Check sheet for the modelled part. Datum: model origin and axes. Units: mm. A direction names the side the tool comes from. Give positions to 0.01 mm unless a question says otherwise; leave off trailing zeros. Write each loop counter-clockwise with the first axis right and the second up, starting at its lowest first coordinate (ties: lowest second). Pieces come first, ordered by that corner, then holes. Notation, with made-up numbers: (6, -2.75) -> (18, -2.75) arc R34 ccw to (18, 31.25) -> close; hole circle Ø2 at (-31.75, -33.75). An arc over 180 degrees is marked (long way). Write each question's results on one line, items separated by ' | '. Start each with the question number.
Autodesk Inventor part; units mm, degrees
ref_plane "YZ Plane" through (0, 0, 0) normal (1, 0, 0) x (0, 1, 0)
ref_plane "XZ Plane" through (0, 0, 0) normal (0, 1, 0) x (-1, 0, 0)
ref_plane "XY Plane" through (0, 0, 0) normal (0, 0, 1) x (1, 0, 0)
sketch "Sketch1" plane through (0, 0, 0) normal (0, 0, 1) x (1, 0, 0)
  line L0 (0, 0) -> (-112.5, 0) construction
  line L1 (-112.5, 0) -> (112.5, 0) construction
  line L2 (0, 0) -> (0, 100) construction
  line L3 (0, 100) -> (0, -100) construction
  line L4 (0, 0) -> (-75, 0) construction
  line L5 (-75, 0) -> (-75, -55) construction
  line L6 (0, 0) -> (75, 0) construction
  line L7 (75, 0) -> (75, -55) construction
  arc A0 (-72.2813, -59.7687) -> (72.2813, -59.7687) centre (0, -15.4013) ccw
  line L8 (-112.5, 0) -> (-112.5, -45)
  line L9 (-102.5, -55) -> (-80.8039, -55)
  line L10 (80.8039, -55) -> (102.5, -55)
  line L11 (112.5, -45) -> (112.5, 0)
  line L12 (-75, 0) -> (-75, 55) construction
  line L13 (75, 0) -> (75, 55) construction
  arc A1 (72.2746, 59.7368) -> (-72.2746, 59.7368) centre (0, 15) ccw
  line L14 (-80.7775, 55) -> (-102.5, 55)
  line L15 (-112.5, 45) -> (-112.5, 0)
  line L16 (80.7775, 55) -> (102.5, 55)
  line L17 (112.5, 45) -> (112.5, 0)
  arc A2 (-102.5, 55) -> (-112.5, 45) centre (-102.5, 45) ccw
  arc A3 (-80.7775, 55) -> (-72.2746, 59.7368) centre (-80.7775, 65) ccw
  arc A4 (72.2746, 59.7368) -> (80.7775, 55) centre (80.7775, 65) ccw
  arc A5 (112.5, 45) -> (102.5, 55) centre (102.5, 45) ccw
  arc A6 (102.5, -55) -> (112.5, -45) centre (102.5, -45) ccw
  arc A7 (80.8039, -55) -> (72.2813, -59.7687) centre (80.8039, -65) ccw
  arc A8 (-72.2813, -59.7687) -> (-80.8039, -55) centre (-80.8039, -65) ccw
  arc A9 (-112.5, -45) -> (-102.5, -55) centre (-102.5, -45) ccw
  line L18 (-72.2746, 59.7368) -> (-61.9878, 53.5577) construction
  line L19 (-61.9878, 53.5577) -> (-58.8982, 58.7011)
  line L20 (-58.8982, 58.7011) -> (-33.1812, 43.2534)
  line L21 (-33.1812, 43.2534) -> (-36.2707, 38.11)
  line L22 (-36.2707, 38.11) -> (-61.9878, 53.5577)
  line L23 (-58.8982, 58.7011) -> (-56.8385, 62.1301)
  line L24 (-56.8385, 62.1301) -> (-31.1215, 46.6823)
  line L25 (-31.1215, 46.6823) -> (-28.0319, 51.8257)
  line L26 (-28.0319, 51.8257) -> (-53.749, 67.2735)
  line L27 (-53.749, 67.2735) -> (-56.8385, 62.1301)
  line L28 (75.9108, 56.2641) -> (66.1713, 49.254) construction
  line L29 (66.1713, 49.254) -> (62.6662, 54.1238) construction
  line L30 (62.6662, 54.1238) -> (38.3174, 36.5986) construction
  line L31 (38.3174, 36.5986) -> (41.8224, 31.7289) construction
  line L32 (41.8224, 31.7289) -> (66.1713, 49.254) construction
  line L33 (62.6662, 54.1238) -> (56.8245, 62.2401) construction
  line L34 (56.8245, 62.2401) -> (60.3296, 57.3703) construction
  line L35 (60.3296, 57.3703) -> (35.9829, 39.842) construction
  line L36 (35.9829, 39.842) -> (32.4779, 44.7118) construction
  line L37 (32.4779, 44.7118) -> (56.8245, 62.2401) construction
  line L38 (-75, -55) -> (-66.4238, -46.6067) construction
  line L39 (-66.4238, -46.6067) -> (-55.2326, -58.0416) construction
  line L40 (-55.2326, -58.0416) -> (-59.4293, -53.7535) construction
  line L41 (-59.4293, -53.7535) -> (-37.9887, -32.7702) construction
  line L42 (-37.9887, -32.7702) -> (-33.792, -37.0583) construction
  line L43 (-55.2326, -58.0416) -> (-33.792, -37.0583) construction
  line L44 (-66.4238, -46.6067) -> (-62.2271, -50.8948) construction
  line L45 (-62.2271, -50.8948) -> (-40.7865, -29.9114) construction
  line L46 (-40.7865, -29.9114) -> (-44.9832, -25.6233) construction
  line L47 (-44.9832, -25.6233) -> (-66.4238, -46.6067) construction
  line L48 (66.1713, -50.8948) -> (57.2172, -64.1547) construction
  line L49 (57.2172, -64.1547) -> (60.3546, -59.0403) construction
  line L50 (60.3546, -59.0403) -> (34.7828, -43.3533) construction
  line L51 (34.7828, -43.3533) -> (31.6454, -48.4676) construction
  line L52 (57.2172, -64.1547) -> (31.6454, -48.4676) construction
  line L53 (66.1713, -50.8948) -> (62.8135, -55.8672) construction
  line L54 (62.8135, -55.8672) -> (37.2417, -40.1802) construction
  line L55 (37.2417, -40.1802) -> (40.3791, -35.0658) construction
  line L56 (0, 100) -> (0, 82)
  line L57 (0, 82) -> (-25, 82)
  line L58 (-30, 82) -> (25, 82)
  line L59 (30, 77) -> (30, 72)
  line L60 (25, 67) -> (-25, 67)
  line L61 (-30, 72) -> (-30, 77)
  arc A10 (-25, 82) -> (-30, 77) centre (-25, 77) ccw
  arc A11 (-30, 72) -> (-25, 67) centre (-25, 72) ccw
  arc A12 (25, 67) -> (30, 72) centre (25, 72) ccw
  arc A13 (30, 77) -> (25, 82) centre (25, 77) ccw
  line L62 (0, -100) -> (0, -82) construction
  line L63 (0, -82) -> (-25, -82)
  line L64 (-30, -82) -> (25, -82)
  line L65 (30, -77) -> (30, -72)
  line L66 (25, -67) -> (-25, -67)
  line L67 (-30, -72) -> (-30, -77)
  arc A14 (-25, -67) -> (-30, -72) centre (-25, -72) ccw
  arc A15 (-30, -77) -> (-25, -82) centre (-25, -77) ccw
  arc A16 (25, -82) -> (30, -77) centre (25, -77) ccw
  arc A17 (30, -72) -> (25, -67) centre (25, -72) ccw
  line L68 (66.1713, -50.8948) -> (40.3791, -35.0658) construction
  line L69 (102.5, 55) -> (102.5, 45) construction
  line L70 (112.5, 45) -> (109.5, 45) construction
  line L71 (107.5, 45) -> (81.5, 45)
  line L72 (79.5, 43) -> (79.5, 42)
  line L73 (81.5, 40) -> (107.5, 40)
  line L74 (109.5, 42) -> (109.5, 43)
  arc A18 (81.5, 45) -> (79.5, 43) centre (81.5, 43) ccw
  arc A19 (79.5, 42) -> (81.5, 40) centre (81.5, 42) ccw
  arc A20 (107.5, 40) -> (109.5, 42) centre (107.5, 42) ccw
  arc A21 (109.5, 43) -> (107.5, 45) centre (107.5, 43) ccw
  line L75 (102.5, -45) -> (102.5, -55) construction
  line L76 (112.5, -45) -> (109.5, -45) construction
  line L77 (107.5, -45) -> (81.5, -45)
  line L78 (79.5, -43) -> (79.5, -42)
  line L79 (81.5, -40) -> (107.5, -40)
  line L80 (109.5, -42) -> (109.5, -43)
  arc A22 (79.5, -43) -> (81.5, -45) centre (81.5, -43) ccw
  arc A23 (81.5, -40) -> (79.5, -42) centre (81.5, -42) ccw
  arc A24 (107.5, -45) -> (109.5, -43) centre (107.5, -43) ccw
  arc A25 (109.5, -42) -> (107.5, -40) centre (107.5, -42) ccw
  line L81 (79.5, -40) -> (79.5, -30) construction
  line L82 (79.5, 40) -> (79.5, 30) construction
  line L83 (74.5, 30) -> (69.5, 30)
  line L84 (64.5, 25) -> (64.5, -25)
  line L85 (69.5, -30) -> (74.5, -30)
  line L86 (79.5, 25) -> (79.5, -25)
  arc A26 (69.5, 30) -> (64.5, 25) centre (69.5, 25) ccw
  arc A27 (64.5, -25) -> (69.5, -30) centre (69.5, -25) ccw
  arc A28 (74.5, -30) -> (79.5, -25) centre (74.5, -25) ccw
  arc A29 (79.5, 25) -> (74.5, 30) centre (74.5, 25) ccw
  line L87 (-102.5, -55) -> (-102.5, -45) construction
  line L88 (-112.5, -45) -> (-109.5, -45) construction
  line L89 (-107.5, -45) -> (-81.5, -45)
  line L90 (-79.5, -43) -> (-79.5, -42)
  line L91 (-81.5, -40) -> (-107.5, -40)
  line L92 (-109.5, -42) -> (-109.5, -43)
  arc A30 (-107.5, -40) -> (-109.5, -42) centre (-107.5, -42) ccw
  arc A31 (-109.5, -43) -> (-107.5, -45) centre (-107.5, -43) ccw
  arc A32 (-81.5, -45) -> (-79.5, -43) centre (-81.5, -43) ccw
  arc A33 (-79.5, -42) -> (-81.5, -40) centre (-81.5, -42) ccw
  line L93 (-102.5, 55) -> (-102.5, 45) construction
  line L94 (-112.5, 45) -> (-109.5, 45) construction
  line L95 (-107.5, 45) -> (-81.5, 45)
  line L96 (-79.5, 43) -> (-79.5, 42)
  line L97 (-81.5, 40) -> (-107.5, 40)
  line L98 (-109.5, 42) -> (-109.5, 43)
  arc A34 (-107.5, 45) -> (-109.5, 43) centre (-107.5, 43) ccw
  arc A35 (-109.5, 42) -> (-107.5, 40) centre (-107.5, 42) ccw
  arc A36 (-81.5, 40) -> (-79.5, 42) centre (-81.5, 42) ccw
  arc A37 (-79.5, 43) -> (-81.5, 45) centre (-81.5, 43) ccw
  line L99 (-79.5, 40) -> (-79.5, 30) construction
  line L100 (-79.5, 25) -> (-79.5, -25) construction
  line L101 (-79.5, -40) -> (-79.5, -30) construction
  line L102 (-74.5, -30) -> (-69.5, -30)
  line L103 (-64.5, -25) -> (-64.5, 25)
  line L104 (-69.5, 30) -> (-74.5, 30)
  line L105 (-79.5, 30) -> (-79.5, -30)
  arc A38 (-74.5, 30) -> (-79.5, 25) centre (-74.5, 25) ccw
  arc A39 (-64.5, 25) -> (-69.5, 30) centre (-69.5, 25) ccw
  arc A40 (-69.5, -30) -> (-64.5, -25) centre (-69.5, -25) ccw
  arc A41 (-79.5, -25) -> (-74.5, -30) centre (-74.5, -25) ccw
  point P0 (112.5, -55)
  point P1 (30, 82)
  point P2 (30, 67)
  point P3 (30, -82)
  point P4 (30, -67)
  point P5 (79.5, 45)
  point P6 (79.5, -45)
  point P7 (64.5, 30)
  point P8 (-79.5, -45)
  point P9 (-79.5, 45)
  point P10 (-64.5, -30)
  dimension "d0" = 112.5
  dimension "d1" = 225
  dimension "d2" = 100
  dimension "d3" = 200
  dimension "d4" = 75
  dimension "d5" = 55
  dimension "d6" = 75
  dimension "d7" = 55
  dimension "d8" = 55
  dimension "d9" = 10
  dimension "d10" = 12
  dimension "d11" = 6
  dimension "d12" = 30
  dimension "d13" = 4
  dimension "d14" = 6
  dimension "d15" = 12
  dimension "d16" = 6
  dimension "d17" = 30
  dimension "d18" = 10
  dimension "d19" = 6
  dimension "d20" = 30
  dimension "d21" = 6
  dimension "d22" = 12
  dimension "d23" = 16
  dimension "d24" = 6
  dimension "d25" = 30
  dimension "d26" = 6
  dimension "d27" = 16
  dimension "d28" = 6
  dimension "d29" = 30
  dimension "d30" = 6
  dimension "d31" = 30
  dimension "d32" = 6
  dimension "d33" = 18
  dimension "d34" = 30
  dimension "d35" = 60
  dimension "d36" = 15
  dimension "d37" = 5
  dimension "d38" = 18
  dimension "d39" = 30
  dimension "d40" = 60
  dimension "d41" = 15
  dimension "d42" = 5
  dimension "d43" = 3
  dimension "d44" = 30
  dimension "d45" = 5
  dimension "d46" = 2
  dimension "d47" = 2
  dimension "d48" = 30
  dimension "d49" = 5
  dimension "d50" = 2
  dimension "d51" = 10
  dimension "d52" = 10
  dimension "d53" = 15
  dimension "d54" = 5
  dimension "d55" = 3
  dimension "d56" = 30
  dimension "d57" = 2
  dimension "d58" = 3
  dimension "d59" = 30
  dimension "d60" = 5
  dimension "d61" = 2
  dimension "d62" = 10
  dimension "d63" = 70
extrude "Extrusion1" add sketch "Sketch1" along normal blind 10 contours A8 L9 A9 L8 L15 A2 L14 A3 A1 A4 L16 A5 L17 L11 A6 L10 A7 A0 | L27 L26 L25 L24 | L19 L20 L21 L22
properties part number "dudukansayapdrone"
Item 1: Mould release check, pull along X, two halves, no side actions. Record for faces 4 (the cylindrical face through (-75.98, -56.24, 4.93)), 5 (the flat face through (95, 45, 5)), 6 (the flat face through (92, -55, 5)): pulls with the +X half, pulls with the -X half, needs draft (parallel to the pull), parting line crosses it, or undercut.
Item 2: Thickness scan on probe 1 along Y at (x, z) = (-2, 6); probe 2 along Y at (x, z) = (-11, 7.5); probe 3 along X at (y, z) = (80, 5.25). Record the ranges inside material, lowest first. Write a range as from..to.
Item 3: Section check D-D on x = 39.5. Record the boundary of the cut face in (y, z), then the cut area to 3 significant figures.
Item 4: Section check C-C on x = -12. Record the boundary of the cut face in (y, z).
Item 5: Section check A-A on x = -92.5. Record the boundary of the cut face in (y, z), then the cut area to 3 significant figures.
Item 6: Set-up check for faces 1 (the cylindrical face through (-28, -81, 5)), 2 (the flat face through (-91, 55, 5)), 3 (the flat face through (91, 55, 5)): record each of +Z, -Z, +X, -X, +Y, -Y from which the full face is reachable in a straight line by a thin tool's end or side.
Item 7: Section check B-B on z = 5.75. Count the separate pieces of the cut face and the enclosed holes in it, then the cut area to 3 significant figures.
Item 8: Depth check by flat-ended pin: pin 1 Ø5 at (x, z) = (-98, 4.5) entering from -Y; pin 2 Ø5.5 at (y, z) = (73.5, 5.5) entering from +X; pin 3 Ø2 at (x, z) = (-15, 5) entering from -Y; pin 4 Ø6 at (x, y) = (67.5, 69) entering from +Z. Enter the tip coordinate at first touch or a pass-through.
Check sheet entries:
1) face 4: pulls with the -X half | face 5: undercut | face 6: needs draft
2) probe 1: y = -100.19..-82, -67..67, 82..99.98 | probe 2: y = -99.5..-82, -67..67, 82..99.29 | probe 3: x = -54.77..-29, 29..54.77
3) outline: (-90.45, 0) -> (90.26, 0) -> (90.26, 10) -> (-90.45, 10) -> close | area: 1,810 mm^2
4) outline: (-99.36, 0) -> (-82, 0) -> (-82, 10) -> (-99.36, 10) -> close; (-67, 0) -> (67, 0) -> (67, 10) -> (-67, 10) -> close; (82, 0) -> (99.15, 0) -> (99.15, 10) -> (82, 10) -> close
5) outline: (-55, 0) -> (-45, 0) -> (-45, 10) -> (-55, 10) -> close; (-40, 0) -> (40, 0) -> (40, 10) -> (-40, 10) -> close; (45, 0) -> (55, 0) -> (55, 10) -> (45, 10) -> close | area: 1,000 mm^2
6) face 1: +Z, -Z | face 2: +Z, -Z, -X, +Y | face 3: +Z, -Z, +X, +Y
7) separate pieces: 1 | enclosed holes: 8 | area: 30,200 mm^2
8) pin 1: stops at y = -55 | pin 2: stops at x = 64.16 | pin 3: stops at y = -99.05 | pin 4: stops at z = 10
